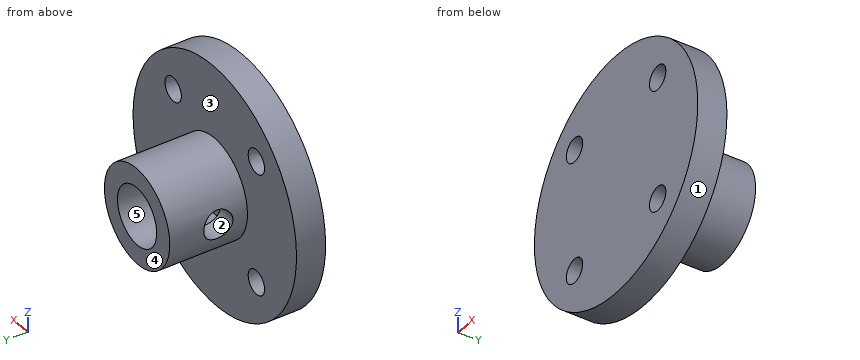
from build123d import *

# Parameters (mm, degrees)
CROQUIS1_R              = 12.5
CROQUIS1_R_2            = 1.25
SALIENTE_EXTRUIR1_DEPTH = 3
SALIENTE_EXTRUIR2_START = 3
CROQUIS1_3_R            = 5
CROQUIS1_3_R_2          = 3
SALIENTE_EXTRUIR2_DEPTH = 8
CROQUIS2_R              = 1.5
CORTAR_EXTRUIR1_DEPTH   = 21.820662814


with BuildPart() as part:
    # Croquis1 → Saliente-Extruir1 (new body)
    with BuildSketch(Plane(origin=(0, 0, 0), x_dir=(1, 0, 0), z_dir=(0, 1, 0))):
        with Locations(Location((0, 0, 0), (0, 0, 270))):
            Circle(CROQUIS1_R)
        with Locations(Location((-6.363961031, 6.363961031, 0), (0, 0, 270))):
            Circle(CROQUIS1_R_2, mode=Mode.SUBTRACT)
        with Locations(Location((6.363961031, 6.363961031, 0), (0, 0, 270))):
            Circle(CROQUIS1_R_2, mode=Mode.SUBTRACT)
        with Locations(Location((6.363961031, -6.363961031, 0), (0, 0, 270))):
            Circle(CROQUIS1_R_2, mode=Mode.SUBTRACT)
        with Locations(Location((-6.363961031, -6.363961031, 0), (0, 0, 270))):
            Circle(CROQUIS1_R_2, mode=Mode.SUBTRACT)
    extrude(amount=SALIENTE_EXTRUIR1_DEPTH)

    # Croquis1<3> → Saliente-Extruir2 (add)
    with BuildSketch(Plane(origin=(0, 0, 0), x_dir=(1, 0, 0), z_dir=(0, 1, 0)).offset(SALIENTE_EXTRUIR2_START)):
        with Locations(Location((0, 0, 0), (0, 0, 270))):
            Circle(CROQUIS1_3_R)
        with Locations(Location((0, 0, 0), (0, 0, 270))):
            Circle(CROQUIS1_3_R_2, mode=Mode.SUBTRACT)
    extrude(amount=SALIENTE_EXTRUIR2_DEPTH)

    # Croquis2 → Cortar-Extruir1 (cut, through all)
    with BuildSketch(Plane(origin=(0, 0, 0), x_dir=(0, 0, -1), z_dir=(1, 0, 0))):
        with Locations((0, 6)):
            Circle(CROQUIS2_R)
    extrude(amount=-CORTAR_EXTRUIR1_DEPTH, mode=Mode.SUBTRACT)


solid = part.part
Design review of the part built by this model. Coordinates are the model's own, in mm. Face numbers are marked on the shaded views. A direction names the side the tool comes from. Round coordinates to 2 decimals unless told otherwise and drop trailing zeros. Write each loop counter-clockwise with the first axis right and the second up, starting at its lowest first coordinate (ties: lowest second). Pieces come first, ordered by that corner, then holes.
Item 1: For the marked faces 4 and 5, list the 3-axis set-ups (+Z, -Z, +X, -X, +Y, -Y) from which the entire face can be reached by the end or side of a thin tool; tool diameter is ignored.
Item 2: Consider section A-A on z = 0. Give the boundary of the cut face in (x, y), and give its area (3 significant figures).
Item 3: Consider section C-C on z = -7.25. Give the boundary of the cut face in (x, y), and give its area (3 significant figures).
Item 4: For pin 1 Ø2 at (x, z) = (8.5, 7) entering from +Y; pin 2 Ø5 at (y, z) = (6, 0) entering from +X; pin 3 Ø1 at (x, y) = (-2, 4.5) entering from -Z, all flat-tipped, find the tip position at first contact; note any pin that passes through.
Item 5: Consider section B-B on x = 5.75. Give the boundary of the cut face in (y, z), and give its area (3 significant figures).
Item 6: Consider section D-D on x = 0. Give the boundary of the cut face in (y, z), and give its area (3 significant figures).
Item 7: Wall thickness on L1, parallel to Z at x = -6.75, y = 2.25; L2, parallel to Z at x = -3.75, y = 5.5; L3, parallel to X at y = 9.25, z = 2.75: over which ranges is each line inside the solid? List them lowest first.
Item 8: Draft analysis for pull direction Y (two halves, no side actions). For the marked faces 1, 2 and 3, state which applies: released by +Y, released by -Y, zero draft, split by the parting line, or undercut.
Check values:
1. face 4: +Z, -Z, +X, -X, +Y
1. face 5: +Y
2. outline: (-12.5, 0) - (12.5, 0) - (12.5, 3) - (5, 3) - (5, 11) - (3, 11) - (3, 3) - (-3, 3) - (-3, 4.5) - (-5, 4.5) - (-5, 3) - (-12.5, 3) - close; (-5, 7.5) - (-3, 7.5) - (-3, 11) - (-5, 11) - close
2. area: 101 mm2
3. outline: (-10.18, 0) - (-7.25, 0) - (-7.25, 3) - (-10.18, 3) - close; (-5.48, 0) - (5.48, 0) - (5.48, 3) - (-5.48, 3) - close; (7.25, 0) - (10.18, 0) - (10.18, 3) - (7.25, 3) - close
3. area: 50.5 mm2
4. pin 1: stops at y = 3
4. pin 2: stops at x = 5
4. pin 3: stops at z = -4.77
5. outline: (0, -11.1) - (3, -11.1) - (3, -7.45) - (0, -7.45) - close; (0, -5.28) - (3, -5.28) - (3, 5.28) - (0, 5.28) - close; (0, 7.45) - (3, 7.45) - (3, 11.1) - (0, 11.1) - close
5. area: 53.5 mm2
6. outline: (0, -12.5) - (3, -12.5) - (3, -5) - (11, -5) - (11, -3) - (3, -3) - (3, 3) - (11, 3) - (11, 5) - (3, 5) - (3, 12.5) - (0, 12.5) - close
6. area: 107 mm2
7. L1: z = -10.52 to -7.55, -5.18 to 5.18, 7.55 to 10.52
7. L2: z = -3.31 to -1.41, 1.41 to 3.31
7. L3: x = -4.18 to -1.2, 1.2 to 4.18
8. face 1: zero draft
8. face 2: undercut
8. face 3: released by +Y
